For this review, take the finished solid that the model builds, in its own axes (mm). Face numbers are marked on the shaded views. A direction names the side the tool comes from. Give positions to 0.01 mm unless a question says otherwise; leave off trailing zeros. Write each loop counter-clockwise with the first axis right and the second up, starting at its lowest first coordinate (ties: lowest second). Pieces come first, ordered by that corner, then holes. Notation, with made-up numbers: (63.25, -6.75) -> (80.25, -6.75) arc R15 ccw to (80.25, 11.25) -> close; hole circle Ø7 at (58.25, 76.5). An arc over 180 degrees is marked (long way). Write item = value, one per line.
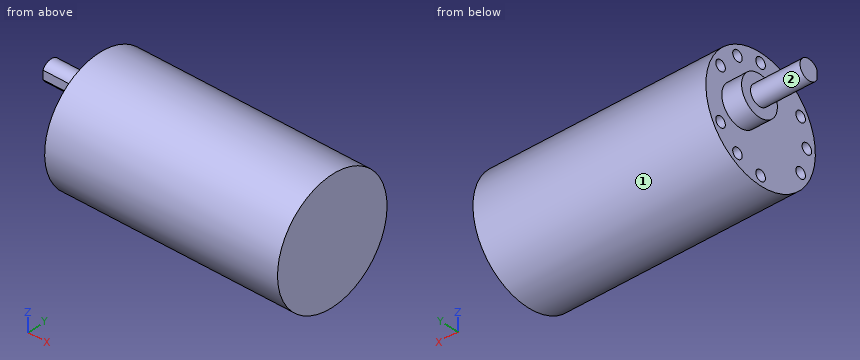
```python
from build123d import *

# Parameters (mm, degrees)
ESQUISSE1_R             = 18.35
BOSS_EXTRU_1_DEPTH      = 70.64
ESQUISSE11_R            = 1.6
ENL_V_MAT_EXTRU_1_DEPTH = 10
ESQUISSE12_R            = 3
BOSS_EXTRU_2_DEPTH      = 21
ESQUISSE13_R            = 6
BOSS_EXTRU_3_DEPTH      = 6
ENL_V_START             = -11.8
ENL_V_MAT_EXTRU_2_DEPTH = 11.8


with BuildPart() as part:
    # Esquisse1 → Boss.-Extru.1 (new body)
    with BuildSketch(Plane(origin=(0, 0, 0), x_dir=(0, 0, -1), z_dir=(1, 0, 0))):
        Circle(ESQUISSE1_R)
    extrude(amount=BOSS_EXTRU_1_DEPTH)

    # Esquisse11 → Enlèv. mat.-Extru.1 (cut)
    with BuildSketch(Plane.ZY):
        with Locations((0, -15.5)):
            Circle(ESQUISSE11_R)
        with Locations((-7.75, -13.423393759)):
            Circle(ESQUISSE11_R)
        with Locations((-15.5, 0)):
            Circle(ESQUISSE11_R)
        with Locations((-13.423393759, 7.75)):
            Circle(ESQUISSE11_R)
        with Locations((-7.75, 13.423393759)):
            Circle(ESQUISSE11_R)
        with Locations((7.75, 13.423393759)):
            Circle(ESQUISSE11_R)
        with Locations((13.423393759, 7.75)):
            Circle(ESQUISSE11_R)
        with Locations((15.5, 0)):
            Circle(ESQUISSE11_R)
        with Locations((7.75, -13.423393759)):
            Circle(ESQUISSE11_R)
    extrude(amount=-ENL_V_MAT_EXTRU_1_DEPTH, mode=Mode.SUBTRACT)

    # Esquisse12 → Boss.-Extru.2 (add)
    with BuildSketch(Plane.ZY):
        with Locations(Location((0, 7, 0), (0, 0, 180))):
            Circle(ESQUISSE12_R)
    extrude(amount=BOSS_EXTRU_2_DEPTH)

    # Esquisse13 → Boss.-Extru.3 (add)
    with BuildSketch(Plane.ZY):
        with Locations(Location((0, 7, 0), (0, 0, 180))):
            Circle(ESQUISSE13_R)
    extrude(amount=BOSS_EXTRU_3_DEPTH)

    # Esquisse14 → Enlèv. mat.-Extru.2 (cut)
    with BuildSketch(Plane.ZY.offset(21).offset(ENL_V_START)):
        with BuildLine():
            Line((-1.307669683, 4.3), (1.307669683, 4.3))
            ThreePointArc((1.307669683, 4.3), (0, 4), (-1.307669683, 4.3))
        make_face()
    extrude(amount=ENL_V_MAT_EXTRU_2_DEPTH, mode=Mode.SUBTRACT)


solid = part.part
```
(1) For pin 1 (5 mm diameter, centred on y = 13.42, z = 7.75, fed in from -X); pin 2 (8 mm diameter, centred on x = 51, z = 4, fed in from -Y); pin 3 (2.5 mm diameter, centred on y = 0, z = 15.5, fed in from -X), all flat-tipped, find the tip position at first contact; note any pin that passes through.
Answers below:
pin_1 = 0
pin_2 = -18.35
pin_3 = 10
(2) To check wall thickness, follow probe 1 along Y at (x, z) = (2.25, 7.75); probe 2 along X at (y, z) = (13, -7.5); probe 3 along X at (y, z) = (6.5, 5.5). State the ranges of each line that lie inside material, in increasing order.
Answers below:
probe_1 = -16.63 to -15.02, -11.82 to 11.82, 15.02 to 16.63
probe_2 = 10 to 70.64
probe_3 = -6 to 70.64
(3) Tool access review of the marked faces 1 and 2: name each direction out of +Z, -Z, +X, -X, +Y, -Y from which nothing blocks a thin tool from reaching the whole face with its end or side.
Answers below:
face_1 = +X, -X
face_2 = -X
(4) Take a section at C-C (x = 56.5). Write out the cut boundary in (y, z).
Answers below:
outline = circle Ø36.7 at (0, 0)
(5) Take a section at B-B (z = 5). Write out the cut boundary in (x, y), plus the area to 3 significant figures.
Answers below:
outline = (-6, 3.68) -> (0, 3.68) -> (0, -17.66) -> (70.64, -17.66) -> (70.64, 17.66) -> (0, 17.66) -> (0, 10.32) -> (-6, 10.32) -> close
area = 2,530 mm^2
(6) Take a section at A-A (x = 1.5). Count the separate pieces of the cut face and the enclosed holes in it, plus the area to 3 significant figures.
Answers below:
separate_pieces = 1
enclosed_holes = 9
area = 985 mm^2
(7) Take a section at D-D (y = -4.5). Write out the cut boundary in (x, z), plus the area to 3 significant figures.
Answers below:
outline = (0, -17.79) -> (70.64, -17.79) -> (70.64, 17.79) -> (0, 17.79) -> close
area = 2,510 mm^2
